For this review, use the dimensioned drawing (mm, ordinates from the lowest corner) and the shaded views. A direction names the side the tool comes from. Coordinates: 2 decimals unless noted, no trailing zeros. Write each loop counter-clockwise with the first axis right and the second up, starting at its lowest first coordinate (ties: lowest second). Pieces come first, ordered by that corner, then holes. Notation, with made-up numbers: (70, -5.5) -> (103, -5.5) arc R22 ccw to (103, 32.5) -> close; hole circle Ø4 at (-33, 60.25). An arc over 180 degrees is marked (long way). Return JSON: item names as keys, results as strings. Group by question number.
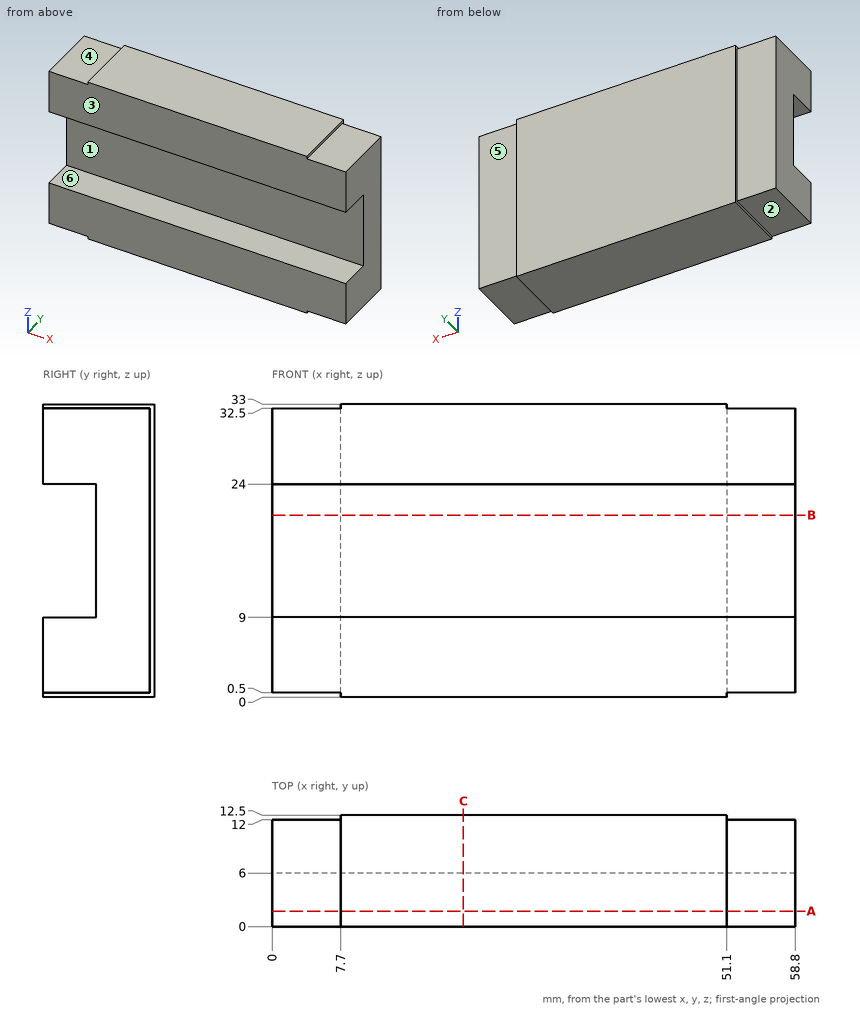
Q1. For P1, Ø1.8, axis at x = 31, y = 4, coming from the -Z side; P2, Ø8.5, axis at x = 3, z = 11.5, coming from the +Y side; P3, Ø4, axis at x = 5, y = 8.5, coming from the +Z side; P4, Ø4, axis at y = 3, z = 20.5, coming from the +X side, all flat-tipped, find the tip position at first contact; note any pin that passes through.
Q2. We need section B-B on z = 20.5. Write out the cut boundary in (x, y), plus the area to 4 significant figures.
Q3. The part is to be moulded in two halves that separate along Z. For the marked faces 1, 2 and 3, say which applies: +Z half, -Z half, draft (parallel to the pull), parting line (faces both ways), or undercut.
Q4. We need section C-C on x = 21.5. Write out the cut boundary in (y, z).
Q5. For the marked faces 4, 5 and 6, list the 3-axis set-ups (+Z, -Z, +X, -X, +Y, -Y) from which the entire face can be reached by the end or side of a thin tool; tool diameter is ignored.
Q6. Wall thickness on L1, parallel to Z at x = 7, y = 2; L2, parallel to Y at x = 3, z = 23.5; L3, parallel to Y at x = 52.5, z = 29.5: over which ranges is each line inside the solid? List them lowest first.
Q7. We need section A-A on y = 1.75. Write out the cut boundary in (x, z), plus the area to 3 significant figures.
Findings below:
{
 "1": {"P1": "stops at z = 0", "P2": "stops at y = 12", "P3": "stops at z = 32.5", "P4": "passes through"},
 "2": {"outline": "(0, 6) -> (58.8, 6) -> (58.8, 12) -> (51.1, 12) -> (51.1, 12.5) -> (7.7, 12.5) -> (7.7, 12) -> (0, 12) -> close", "area": "374.5 mm^2"},
 "3": {"face 1": "undercut", "face 2": "-Z half", "face 3": "draft"},
 "4": {"outline": "(0, 0) -> (12.5, 0) -> (12.5, 33) -> (0, 33) -> (0, 24) -> (6, 24) -> (6, 9) -> (0, 9) -> close"},
 "5": {"face 4": "+Z, -X, +Y, -Y", "face 5": "+Z, -Z, +X, +Y", "face 6": "+X, -X, -Y"},
 "6": {"L1": "z = 0.5 to 9, 24 to 32.5", "L2": "y = 6 to 12", "L3": "y = 0 to 12"},
 "7": {"outline": "(0, 0.5) -> (7.7, 0.5) -> (7.7, 0) -> (51.1, 0) -> (51.1, 0.5) -> (58.8, 0.5) -> (58.8, 9) -> (0, 9) -> close; (0, 24) -> (58.8, 24) -> (58.8, 32.5) -> (51.1, 32.5) -> (51.1, 33) -> (7.7, 33) -> (7.7, 32.5) -> (0, 32.5) -> close", "area": "1,040 mm^2"}
}
